Could you check a few things on this model? Use its own coordinates, in mm. A direction names the side the tool comes from. Coordinates: 2 decimals unless noted, no trailing zeros. Order: outer loops, then holes, each group sorted by start corner. A loop starts at its lowest first (then second) coordinate and runs counter-clockwise, first axis right, second up. Notation, with made-up numbers: (-0.5, 42) -> (36.5, 42) arc R23 ccw to (36.5, 61) -> close; hole circle Ø1 at (82, 6.5). An arc over 180 degrees is marked (long way). Use a Markdown table: item, result. Add a question column.
1) If we section it at D-D (y = 35): Write out the boundary of the cut face in (x, z).
2) If we section it at C-C (z = 19.25): Give the number of separate pieces and of enclosed holes in the cut face, plus the area to 3 significant figures.
3) If we section it at A-A (y = 0): Write out the boundary of the cut face in (x, z).
4) If we section it at B-B (z = -0.75): Write out the boundary of the cut face in (x, y).
5) Will these pins go through, and if not, where does the flat tip stop? pin 1 Ø12 at (x, z) = (-10, 4.5) entering from -Y; pin 2 Ø10 at (x, z) = (-8.5, 4) entering from +Y; pin 3 Ø3 at (y, z) = (32.5, 13.5) entering from -X.
6) Thinking about a two-plate mould opening in X: for faces 1 (the cylindrical face through (63.006, -34.249, 12.36)), 2 (the flat face through (26, 15, 22.5)), which applies, +X half, -X half, draft (parallel to the pull), parting line (faces both ways), or undercut?
7) Which directions (+Z, -Z, +X, -X, +Y, -Y) give clear straight access to the entire face, cutting with the end or side of a thin tool? Please do faces 3 (the flat face through (35, -61, 22.5)), 4 (the cylindrical face through (1.15, -72.22, 12.36)).
8) If I drill on L1, parallel to Y at x = -26, z = 12.75; L2, parallel to Z at x = -19, y = 40.5; L3, parallel to X at y = -50.5, z = 20.5, over which ranges is the centre line in solid material (lowest first)? Write a range as [from, to].
```python
from build123d import *

# Parameters (mm, degrees)
F2_R     = 75
F3_DEPTH = 2.5
F4_R     = 2.5
F5_DEPTH = 20


with BuildPart() as f3:
    # F2 (on Top) → F3 (new body, symmetric)
    with BuildSketch(Plane.XY):
        Circle(F2_R)
    extrude(amount=F3_DEPTH, both=True)

    # F4 (on face) → F5 (join)
    with BuildSketch(Plane.XY.offset(2.5)):
        with Locations((-15, 25.9807621135)):
            Circle(F4_R)
        with Locations((0, 70)):
            Circle(F4_R)
        with Locations((-18.1173331572, 67.6148078402)):
            Circle(F4_R)
        with Locations((-35, 60.6217782649)):
            Circle(F4_R)
        with Locations((-49.4974746831, 49.4974746831)):
            Circle(F4_R)
        with Locations((-60.6217782649, 35)):
            Circle(F4_R)
        with Locations((-67.6148078402, 18.1173331572)):
            Circle(F4_R)
        with Locations((-70, 0)):
            Circle(F4_R)
        with Locations((-67.6148078402, -18.1173331572)):
            Circle(F4_R)
        with Locations((-60.6217782649, -35)):
            Circle(F4_R)
        with Locations((-49.4974746831, -49.4974746831)):
            Circle(F4_R)
        with Locations((-35, -60.6217782649)):
            Circle(F4_R)
        with Locations((-18.1173331572, -67.6148078402)):
            Circle(F4_R)
        with Locations((0, -70)):
            Circle(F4_R)
        with Locations((18.1173331572, -67.6148078402)):
            Circle(F4_R)
        with Locations((35, -60.6217782649)):
            Circle(F4_R)
        with Locations((49.4974746831, -49.4974746831)):
            Circle(F4_R)
        with Locations((60.6217782649, -35)):
            Circle(F4_R)
        with Locations((67.6148078402, -18.1173331572)):
            Circle(F4_R)
        with Locations((70, 0)):
            Circle(F4_R)
        with Locations((67.6148078402, 18.1173331572)):
            Circle(F4_R)
        with Locations((60.6217782649, 35)):
            Circle(F4_R)
        with Locations((49.4974746831, 49.4974746831)):
            Circle(F4_R)
        with Locations((35, 60.6217782649)):
            Circle(F4_R)
        with Locations((18.1173331572, 67.6148078402)):
            Circle(F4_R)
        with Locations((-25.9807621135, 15)):
            Circle(F4_R)
        with Locations((-30, 0)):
            Circle(F4_R)
        with Locations((-25.9807621135, -15)):
            Circle(F4_R)
        with Locations((-15, -25.9807621135)):
            Circle(F4_R)
        with Locations((0, -30)):
            Circle(F4_R)
        with Locations((15, -25.9807621135)):
            Circle(F4_R)
        with Locations((25.9807621135, -15)):
            Circle(F4_R)
        with Locations((30, 0)):
            Circle(F4_R)
        with Locations((25.9807621135, 15)):
            Circle(F4_R)
        with Locations((15, 25.9807621135)):
            Circle(F4_R)
        with Locations((0, 30)):
            Circle(F4_R)
    extrude(amount=F5_DEPTH)


solid = f3.part
```
Answer sheet:
| question | item | result |
|---|---|---|
| 1 | outline | (-66.33, -2.5) -> (66.33, -2.5) -> (66.33, 2.5) -> (63.12, 2.5) -> (63.12, 22.5) -> (58.12, 22.5) -> (58.12, 2.5) -> (-58.12, 2.5) -> (-58.12, 22.5) -> (-63.12, 22.5) -> (-63.12, 2.5) -> (-66.33, 2.5) -> close |
| 2 | separate pieces | 36 |
| 2 | enclosed holes | 0 |
| 2 | area | 707 mm2 |
| 3 | outline | (-75, -2.5) -> (75, -2.5) -> (75, 2.5) -> (72.5, 2.5) -> (72.5, 22.5) -> (67.5, 22.5) -> (67.5, 2.5) -> (32.5, 2.5) -> (32.5, 22.5) -> (27.5, 22.5) -> (27.5, 2.5) -> (-27.5, 2.5) -> (-27.5, 22.5) -> (-32.5, 22.5) -> (-32.5, 2.5) -> (-67.5, 2.5) -> (-67.5, 22.5) -> (-72.5, 22.5) -> (-72.5, 2.5) -> (-75, 2.5) -> close |
| 4 | outline | circle Ø150 at (0, 0) |
| 5 | pin 1 | y = -74.87 |
| 5 | pin 2 | y = 74.91 |
| 5 | pin 3 | x = -62.91 |
| 6 | face 1 | undercut |
| 6 | face 2 | draft |
| 7 | face 3 | +Z, +X, -X, +Y, -Y |
| 7 | face 4 | +Z |
| 8 | L1 | [-17.5, -12.5], [12.5, 17.5] |
| 8 | L2 | [-2.5, 2.5] |
| 8 | L3 | [-51.79, -47.21], [47.21, 51.79] |
